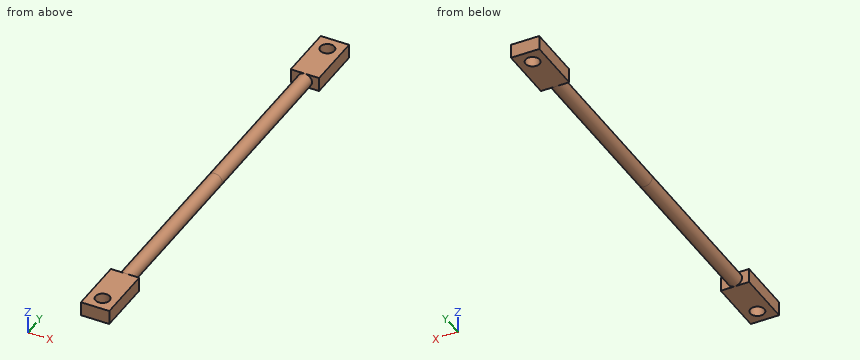
from build123d import *

# Parameters (mm, degrees)
SKETCH1_R           = 1.5875
BOSS_EXTRUDE1_DEPTH = 38.1
SKETCH2_W           = 6.35
SKETCH2_H           = 3.175
BOSS_EXTRUDE2_DEPTH = 12.7
SKETCH3_R           = 1.5875
CUT_EXTRUDE1_DEPTH  = 51.998051433


with BuildPart() as part:
    # Sketch1 → Boss-Extrude1 (new body)
    with BuildSketch(Plane(origin=(0, 0, 0), x_dir=(1, 0, 0), z_dir=(0, 1, 0))):
        with Locations(Location((0, 0, 0), (0, 0, 90))):
            Circle(SKETCH1_R)
    boss_extrude1 = extrude(amount=BOSS_EXTRUDE1_DEPTH)

    # Sketch2 → Boss-Extrude2 (add)
    with BuildSketch(Plane(origin=(0, 38.1, 0), x_dir=(1, 0, 0), z_dir=(0, 1, 0))):
        Rectangle(SKETCH2_W, SKETCH2_H)
    boss_extrude2 = extrude(amount=BOSS_EXTRUDE2_DEPTH)

    # Sketch3 → Cut-Extrude1 (cut, through all)
    with BuildSketch(Plane(origin=(0, 0, -1.5875), x_dir=(-1, 0, 0), z_dir=(0, 0, -1))):
        with Locations((0, 47.625)):
            Circle(SKETCH3_R)
    cut_extrude1 = extrude(amount=-CUT_EXTRUDE1_DEPTH, mode=Mode.SUBTRACT)

    # Mirror1: Boss-Extrude1, Boss-Extrude2, Cut-Extrude1 across plane
    add(boss_extrude1.mirror(Plane.ZX))
    add(boss_extrude2.mirror(Plane.ZX))
    add(cut_extrude1.mirror(Plane.ZX), mode=Mode.SUBTRACT)


solid = part.part
Here's how the part is built. I have some questions about the finished solid (model axes, mm). Coordinates: 2 decimals unless noted, no trailing zeros. Order: outer loops, then holes, each group sorted by start corner. A loop starts at its lowest first (then second) coordinate and runs counter-clockwise, first axis right, second up.
Item 1: For P1, Ø2, axis at x = 1.5, y = -11.5, coming from the +Z side; P2, Ø2.5, axis at x = 0, y = 47.625, coming from the +Z side, each with a flat end and sliding along its axis, tell me the tip position at first contact or that it passes through.
Result sheet:
P1: stops at z = 1.51
P2: passes through
Item 2: If we section it at B-B on y = 17: List the corners of the cut face in (x, z) for me (1 decimal).
Result sheet:
outline: circle Ø3.2 at (0, 0)
Item 3: If we section it at A-A on z = 0: List the corners of the cut face in (x, y) for me (1 decimal), plus the area to 3 significant figures.
Result sheet:
outline: (-3.2, -50.8) - (3.2, -50.8) - (3.2, -38.1) - (1.6, -38.1) - (1.6, 38.1) - (3.2, 38.1) - (3.2, 50.8) - (-3.2, 50.8) - (-3.2, 38.1) - (-1.6, 38.1) - (-1.6, -38.1) - (-3.2, -38.1) - close; hole circle Ø3.2 at (0, -47.6); hole circle Ø3.2 at (0, 47.6)
area: 387 mm2
Item 4: I need wall thicknesses on line 1 (Y direction, x = 0, z = 0.45); line 2 (Y direction, x = 0.25, z = -0.7); line 3 (Y direction, x = -2.25, z = 0.35). Which ranges of each line are inside material? Lowest first, please.
Result sheet:
line 1: y = -50.8 to -49.21, -46.04 to 46.04, 49.21 to 50.8
line 2: y = -50.8 to -49.19, -46.06 to 46.06, 49.19 to 50.8
line 3: y = -50.8 to -38.1, 38.1 to 50.8
